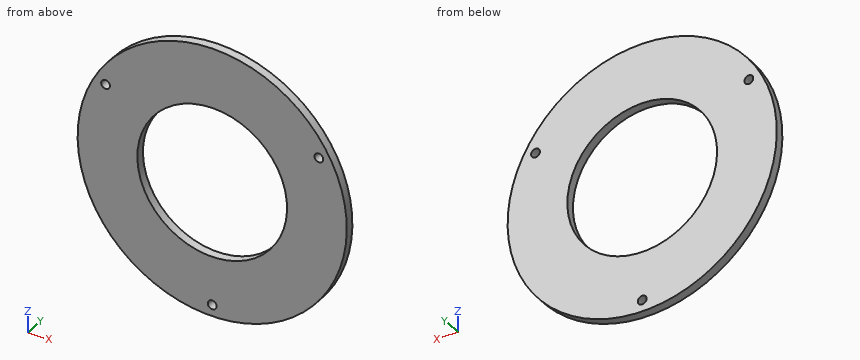
from build123d import *

# Parameters (mm, degrees)
SKETCH1_R           = 97.028
BOSS_EXTRUDE1_DEPTH = 6.35
SKETCH2_R           = 3.175
CUT_EXTRUDE1_DEPTH  = 138.365163226
SKETCH3_R           = 53.975
CUT_EXTRUDE2_DEPTH  = 138.365163226


with BuildPart() as part:
    # Sketch1 → Boss-Extrude1 (new body)
    with BuildSketch(Plane(origin=(0, 0, 0), x_dir=(1, 0, 0), z_dir=(0, 1, 0))):
        with Locations(Location((0, 0, 0), (0, 0, 270))):
            Circle(SKETCH1_R)
    extrude(amount=BOSS_EXTRUDE1_DEPTH)

    # Sketch2 → Cut-Extrude1 (cut, through all)
    with BuildSketch(Plane(origin=(0, 6.35, 0), x_dir=(1, 0, 0), z_dir=(0, 1, 0))):
        with Locations(Location((0, 88.773, 0), (0, 0, 270))):
            Circle(SKETCH2_R)
        with Locations(Location((76.87967317, -44.3865, 0), (0, 0, 270))):
            Circle(SKETCH2_R)
        with Locations(Location((-76.87967317, -44.3865, 0), (0, 0, 270))):
            Circle(SKETCH2_R)
    extrude(amount=-CUT_EXTRUDE1_DEPTH, mode=Mode.SUBTRACT)

    # Sketch3 → Cut-Extrude2 (cut, through all)
    with BuildSketch(Plane(origin=(0, 6.35, 0), x_dir=(1, 0, 0), z_dir=(0, 1, 0))):
        with Locations(Location((0, 0, 0), (0, 0, 270))):
            Circle(SKETCH3_R)
    extrude(amount=-CUT_EXTRUDE2_DEPTH, mode=Mode.SUBTRACT)


solid = part.part
Model file for the job. Use its own axes, mm. Give positions to 0.01 mm unless a question says otherwise; leave off trailing zeros. Write each loop counter-clockwise with the first axis right and the second up, starting at its lowest first coordinate (ties: lowest second). Pieces come first, ordered by that corner, then holes. Notation, with made-up numbers: M -30.5,74 L 25.5,74 A25 cw 25.5,109 Z; hole C -35,-2.75 d7. An arc over 180 degrees is marked long. One line per item, written item: value. Start each with the question number.
Q1. Drop flat-ended pins along their axis: pin 1 Ø4 at (x, z) = (76.88, 44.39) entering from -Y; pin 2 Ø3 at (x, y) = (-48, 2) entering from -Z. Give the stop position or say it passes through.
Q2. Probe probe 1 along X at (y, z) = (3.5, -1); probe 2 along Z at (x, y) = (-2, 4.75); probe 3 along X at (y, z) = (0.5, 10). List the from-to ranges inside material, lowest first. Write a range as [from, to].
Q3. Saw through at C-C, the plane x = 29. Write the cut outline in (y, z), plus the area to 3 significant figures.
Q4. Saw through at B-B, the plane z = 0. Write the cut outline in (x, y) (3 decimals), plus the area to 3 significant figures.
Q5. Saw through at D-D, the plane y = 1.5. State how many separate pieces and enclosed holes the cut face has, plus the area to 3 significant figures.
Q6. Saw through at A-A, the plane x = 0. Write the cut outline in (y, z) (3 decimals), plus the area to 3 significant figures.
Output values:
1. pin 1: passes through
1. pin 2: stops at z = -85.16
2. probe 1: x = [-97.02, -53.97], [53.97, 97.02]
2. probe 2: z = [-97.01, -91.24], [-86.31, -53.94], [53.94, 97.01]
2. probe 3: x = [-96.51, -53.04], [53.04, 96.51]
3. outline: M 0,-92.59 L 6.35,-92.59 L 6.35,-45.52 L 0,-45.52 Z; M 0,45.52 L 6.35,45.52 L 6.35,92.59 L 0,92.59 Z
3. area: 598 mm²
4. outline: M -97.028,0 L -53.975,0 L -53.975,6.35 L -97.028,6.35 Z; M 53.975,0 L 97.028,0 L 97.028,6.35 L 53.975,6.35 Z
4. area: 547 mm²
5. separate pieces: 1
5. enclosed holes: 4
5. area: 20,300 mm²
6. outline: M 0,-97.028 L 6.35,-97.028 L 6.35,-91.948 L 0,-91.948 Z; M 0,-85.598 L 6.35,-85.598 L 6.35,-53.975 L 0,-53.975 Z; M 0,53.975 L 6.35,53.975 L 6.35,97.028 L 0,97.028 Z
6. area: 506 mm²
